from build123d import *

# Parameters (mm, degrees)
F1_DEPTH = 15


with BuildPart() as f1:
    # F0 (on Top) → F1 (new body)
    with BuildSketch(Plane.XY):
        Polygon((0, 2.7), (0, 0), (14.5, 0), (14.5, 2.7), (9.5, 2.7), (9.5, 5.9), (19.5, 5.9), (-5, 105.9), (-5, 5.9), (5, 5.9), (5, 2.7), align=None)
        Polygon((16.87268, 9.9), (-3.4, 9.9), (-3.4, 23.06697), (-3.4, 24.3), (-3, 24.5), (-2.6, 24.5), (-1.8, 24.3), (11.45068, 24.3), (12.25068, 24.5), (12.65068, 24.5), (13.745434, 23.952623), align=None, mode=Mode.SUBTRACT)
        Polygon((8.981001, 39.5), (9.70998, 39.135511), (13.05068, 25.5), (12.65068, 25.3), (12.25068, 25.3), (11.45068, 25.5), (-1.8, 25.5), (-2.6, 25.3), (-3, 25.3), (-3.4, 25.5), (-3.4, 26.733285), (-3.4, 39.299999), (-2.998656, 39.5), (-2.598656, 39.5), (-1.798656, 39.3), (7.781001, 39.3), (8.581001, 39.5), align=None, mode=Mode.SUBTRACT)
        Polygon((5.306001, 54.5), (6.041044, 54.132479), (9.381001, 40.5), (8.981001, 40.3), (8.581001, 40.3), (7.781001, 40.5), (-1.8, 40.5), (-2.6, 40.3), (-3, 40.3), (-3.4, 40.466429), (-3.4, 54.3), (-3, 54.5), (-2.6, 54.5), (-1.8, 54.3), (4.106001, 54.3), (4.906001, 54.5), align=None, mode=Mode.SUBTRACT)
        Polygon((2.366001, 66.5), (3.101044, 66.132479), (5.706001, 55.5), (5.306001, 55.3), (4.906001, 55.3), (4.106001, 55.5), (-1.8, 55.5), (-2.6, 55.3), (-3, 55.3), (-3.4, 55.5), (-3.4, 66.3), (-3, 66.5), (-2.6, 66.5), (-1.8, 66.3), (1.166001, 66.3), (1.966001, 66.5), align=None, mode=Mode.SUBTRACT)
        Polygon((-3.4, 75.38324), (-3.4, 92.645632), (0.804118, 75.485968), (1.518031, 72.593754), (2.766001, 67.5), (2.366001, 67.3), (1.966001, 67.3), (1.166001, 67.5), (-1.8, 67.5), (-2.6, 67.3), (-3, 67.3), (-3.4, 67.5), (-3.4, 72.41676), align=None, mode=Mode.SUBTRACT)
    extrude(amount=F1_DEPTH)


solid = f1.part
Model file for the job. Use its own axes, mm. A direction names the side the tool comes from. Round coordinates to 2 decimals unless told otherwise and drop trailing zeros. Loops run counter-clockwise (first coordinate to the right, second up) from the corner with the lowest first, then second, coordinate; pieces in that order, holes last. Notation, with made-up numbers: (88.5, 80) -> (138.5, 80) arc R10 cw to (138.5, 94) -> close; hole circle Ø1 at (85, -37.75). An arc over 180 degrees is marked (long way). Answer as CSV lines item,"result". Start each with the question number.
1) Slice it at B-B (y = 51). List the corners of the cut face in (x, z), plus the area to 3 significant figures.
2) Pin check, flat tips, straight feed: P1, Ø10, axis at x = 2, y = 67, coming from the -Z side; P2, Ø2, axis at y = 36, z = 4, coming from the +X side; P3, Ø1.6, axis at y = 4.5, z = 8.5, coming from the +X side; P4, Ø0.8, axis at y = 1, z = 4.5, coming from the -X side. Stop position of each tip, or through.
3) Slice it at C-C (z = 4). State how many separate pieces and enclosed holes the cut face has, plus the area to 3 significant figures.
4) Mould opens along Y. For faces 4 (the face through (-5, 57, 7)), 5 (the face through (7, 0, 7)), 6 (the face through (7.69, 47.41, 7.4)), 7 (the face through (7, 9.9, 7)) say: +Y half, -Y half, draft (parallel to the pull), parting line (faces both ways), or undercut.
5) Probe line 1 along X through (y, z) = (89, 14.25); line 2 along X through (y, z) = (83.5, 8.5); line 3 along X through (y, z) = (94, 13.75). List the from-to ranges inside material, lowest first.
6) Tool access for faces 1 (the face through (12, 2.7, 7)), 2 (the face through (0, 5.9, 7)), 3 (the face through (2.133, 70.083, 7.395)): list every direction of +Z, -Z, +X, -X, +Y, -Y with a clear straight run to the whole face (end or side of a thin tool).
7) Slice it at A-A (x = 15.75). List the corners of the cut face in (y, z).
Filled in:
1,outline,"(-5, 0) -> (-3.4, 0) -> (-3.4, 15) -> (-5, 15) -> close; (6.81, 0) -> (8.45, 0) -> (8.45, 15) -> (6.81, 15) -> close"
1,area,"48.6 mm2"
2,P1,"stops at z = 0"
2,P2,"stops at x = 12.37"
2,P3,"stops at x = 9.5"
2,P4,"stops at x = 0"
3,separate pieces,"1"
3,enclosed holes,"5"
3,area,"488 mm2"
4,face 4,"draft"
4,face 5,"-Y half"
4,face 6,"undercut"
4,face 7,"undercut"
5,line 1,"x = -5 to -3.4, -2.51 to -0.86"
5,line 2,"x = -5 to -3.4, -1.16 to 0.49"
5,line 3,"x = -5 to -2.08"
6,face 1,"+Z, -Z, +X"
6,face 2,"+Z, -Z, -X"
6,face 3,"+Z, -Z"
7,outline,"(5.9, 0) -> (9.9, 0) -> (9.9, 15) -> (5.9, 15) -> close; (14.94, 0) -> (21.21, 0) -> (21.21, 15) -> (14.94, 15) -> close"
